```python
from build123d import *

# Parameters (mm, degrees)
CSK_FOR_ST6_3_CROSS_RECESSED_CTSK_HEAD_T_D           = 6.5
CSK_FOR_ST6_3_CROSS_RECESSED_CTSK_HEAD_T_CSINK_D     = 12.6
CSK_FOR_ST6_3_CROSS_RECESSED_CTSK_HEAD_T_CSINK_ANGLE = 90
CSK_FOR_ST6_3_CROSS_RECESSED_CTSK_HE_2_D             = 6.5
CSK_FOR_ST6_3_CROSS_RECESSED_CTSK_HE_2_CSINK_D       = 12.6
CSK_FOR_ST6_3_CROSS_RECESSED_CTSK_HE_2_CSINK_ANGLE   = 90
SKETCH9_R                                            = 1.25
CUT_EXTRUDE1_DEPTH                                   = 50
SKETCH9_3_R                                          = 1.25
CUT_EXTRUDE2_DEPTH                                   = 50
SKETCH9_4_R                                          = 1.25
CUT_EXTRUDE3_DEPTH                                   = 50
SKETCH9_5_R                                          = 1.25
CUT_EXTRUDE4_DEPTH                                   = 50
SKETCH9_7_R                                          = 1.25
CUT_EXTRUDE5_DEPTH                                   = 50
SKETCH9_8_R                                          = 1.25
CUT_EXTRUDE6_DEPTH                                   = 50


with BuildPart() as part:
    # Sketch1 → Revolve1 (revolve)
    with BuildSketch(Plane.XY):
        Polygon((0, 0), (40.5, 0), (40.5, -20), (-13.5, -20), align=None)
    revolve(axis=Axis((40.5, 11.538552748, 0), (0, -1, 0)))

    # CSK for ST6.3 Cross recessed CTSK head t (through all)
    with Locations(Plane(origin=(0, 0, 0), x_dir=(1, 0, 0), z_dir=(0, 1, 0))):
        with Locations((17.07072808, -13.455101055), (63.836068925, -13.508911829), (40.5, 27.017966747)):
            CounterSinkHole(CSK_FOR_ST6_3_CROSS_RECESSED_CTSK_HEAD_T_D / 2, CSK_FOR_ST6_3_CROSS_RECESSED_CTSK_HEAD_T_CSINK_D / 2, counter_sink_angle=CSK_FOR_ST6_3_CROSS_RECESSED_CTSK_HEAD_T_CSINK_ANGLE)

    # CSK for ST6.3 Cross recessed CTSK he 2 (through all)
    with Locations(Plane(origin=(0, 0, 0), x_dir=(1, 0, 0), z_dir=(0, 1, 0))):
        with Locations((17.117314098, 13.517966747), (63.882685902, 13.535897721), (40.5, -26.982033253)):
            CounterSinkHole(CSK_FOR_ST6_3_CROSS_RECESSED_CTSK_HE_2_D / 2, CSK_FOR_ST6_3_CROSS_RECESSED_CTSK_HE_2_CSINK_D / 2, counter_sink_angle=CSK_FOR_ST6_3_CROSS_RECESSED_CTSK_HE_2_CSINK_ANGLE)

    # Sketch9 → Cut-Extrude1 (cut)
    with BuildSketch(Plane.XZ.offset(20)):
        with Locations((89.719555543, -8.799735913)):
            Circle(SKETCH9_R)
    extrude(amount=-CUT_EXTRUDE1_DEPTH, mode=Mode.SUBTRACT)

    # Sketch9<3> → Cut-Extrude2 (cut)
    with BuildSketch(Plane.XZ.offset(20)):
        with Locations((72.730572619, 38.225517507)):
            Circle(SKETCH9_3_R)
    extrude(amount=-CUT_EXTRUDE2_DEPTH, mode=Mode.SUBTRACT)

    # Sketch9<4> → Cut-Extrude3 (cut)
    with BuildSketch(Plane.XZ.offset(20)):
        with Locations((23.511017076, 47.02525342)):
            Circle(SKETCH9_4_R)
    extrude(amount=-CUT_EXTRUDE3_DEPTH, mode=Mode.SUBTRACT)

    # Sketch9<5> → Cut-Extrude4 (cut)
    with BuildSketch(Plane.XZ.offset(20)):
        with Locations((-8.719555543, 8.799735913)):
            Circle(SKETCH9_5_R)
    extrude(amount=-CUT_EXTRUDE4_DEPTH, mode=Mode.SUBTRACT)

    # Sketch9<7> → Cut-Extrude5 (cut)
    with BuildSketch(Plane.XZ.offset(20)):
        with Locations((8.269427381, -38.225517507)):
            Circle(SKETCH9_7_R)
    extrude(amount=-CUT_EXTRUDE5_DEPTH, mode=Mode.SUBTRACT)

    # Sketch9<8> → Cut-Extrude6 (cut)
    with BuildSketch(Plane.XZ.offset(20)):
        with Locations((57.488982924, -47.02525342)):
            Circle(SKETCH9_8_R)
    extrude(amount=-CUT_EXTRUDE6_DEPTH, mode=Mode.SUBTRACT)


solid = part.part
```
Can you work these out from the model? Positions are in its coordinate system, mm. Round coordinates to 2 decimals unless told otherwise and drop trailing zeros. Order: outer loops, then holes, each group sorted by start corner. A loop starts at its lowest first (then second) coordinate and runs counter-clockwise, first axis right, second up. Notation, with made-up numbers: (-20.75, 47.25) -> (38.25, 47.25) arc R11 ccw to (38.25, 58.25) -> close; hole circle Ø3 at (26, -34.75). An arc over 180 degrees is marked (long way). Return JSON: item names as keys, results as strings. Group by question number.
1. If we section it at C-C, the plane y = -8.75: Write out the boundary of the cut face in (x, z).
2. If we section it at B-B, the plane y = -18.5: Count the separate pieces of the cut face and the enclosed holes in it, then the cut area to 3 significant figures.
3. I need wall thicknesses on line 1 (Z direction, x = 38, y = -16.5); line 2 (Z direction, x = 17, y = -17.75); line 3 (X direction, y = -19, z = 12.5). Which ranges of each line are inside material? Lowest first, please. Write a range as [from, to].
4. If we section it at A-A, the plane x = 40.5: Write out the boundary of the cut face in (y, z).
5. If we section it at D-D, the plane z = 0: Write out the boundary of the cut face in (x, y).
6. Will these pins go through, and if not, where does the flat tip stop? pin 1 (4 mm diameter, centred on y = -12.5, z = -20, fed in from +X); pin 2 (4 mm diameter, centred on x = 8.27, z = -38.23, fed in from -Y); pin 3 (5 mm diameter, centred on x = 14, y = -9.5, fed in from +Z); pin 4 (1 mm diameter, centred on x = 79, y = -11, fed in from -Z).
7. We'd pull the mould along Z, two halves only. Please class faces 1 (the face through (43.895, -2.902, 26.833)), 2 (the face through (2.48, -0.97, 15.76)), 3 (the face through (40, -20, -1)): released by +Z, released by -Z, zero draft, split by the parting line, or undercut.
Output values:
{
 "1": {"outline": "circle Ø92.81 at (40.5, 0); hole circle Ø6.5 at (17.07, 13.46); hole circle Ø6.5 at (17.12, -13.52); hole circle Ø6.5 at (40.5, -27.02); hole circle Ø6.5 at (40.5, 26.98); hole circle Ø6.5 at (63.84, 13.51); hole circle Ø6.5 at (63.88, -13.54)"},
 "2": {"separate pieces": "1", "enclosed holes": "12", "area": "8,590 mm²"},
 "3": {"line 1": "[-51.58, -29.09], [-24.94, 24.91], [29.06, 51.58]", "line 2": "[-46.93, -16.77], [-10.27, 10.21], [16.7, 46.93]", "line 3": "[-11.34, 13.96], [20.18, 60.75], [66.93, 92.34]"},
 "4": {"outline": "(-20, -54) -> (0, -40.5) -> (0, -33.32) -> (-3.05, -30.27) -> (-20, -30.27) -> close; (-20, -23.77) -> (-3.05, -23.77) -> (0, -20.72) -> (0, 20.68) -> (-3.05, 23.73) -> (-20, 23.73) -> close; (-20, 30.23) -> (-3.05, 30.23) -> (0, 33.28) -> (0, 40.5) -> (-20, 54) -> close"},
 "5": {"outline": "(-13.5, -20) -> (94.5, -20) -> (81, 0) -> (0, 0) -> close"},
 "6": {"pin 1": "x = 86.86", "pin 2": "y = -20", "pin 3": "z = 41.28", "pin 4": "z = -29.41"},
 "7": {"face 1": "undercut", "face 2": "split by the parting line", "face 3": "zero draft"}
}
